from build123d import *

# Parameters (mm, degrees)
SKETCH_W        = 34
SKETCH_H        = 30
PAD_DEPTH       = 22
SKETCH001_R     = 5.5
POCKET_DEPTH    = 30.001
SKETCH002_R     = 2
POCKET001_DEPTH = 22.001
CHAMFER_SIZE    = 3
SKETCH003_R     = 7.5
POCKET002_DEPTH = 24
POCKET003_DEPTH = 3.5


with BuildPart() as part:
    # Sketch → Pad (new body)
    with BuildSketch(Plane.XY):
        with Locations((17, 15)):
            Rectangle(SKETCH_W, SKETCH_H)
    extrude(amount=PAD_DEPTH)

    # Sketch001 (on Face1 of Pad) → Pocket (cut, through all)
    with BuildSketch(Plane.XZ):
        with Locations((17, 11)):
            Circle(SKETCH001_R)
        with BuildLine():
            ThreePointArc((17, 22), (6.777476, 15.062019), (9.450166, 3))
            Line((0, 3), (9.450166, 3))
            Line((0, 22), (0, 3))
            Line((17, 22), (0, 22))
        make_face()
        with BuildLine():
            ThreePointArc((24.549834, 3), (27.222524, 15.062019), (17, 22))
            Line((17, 22), (34, 22))
            Line((34, 22), (34, 3))
            Line((34, 3), (24.549834, 3))
        make_face()
    extrude(amount=-POCKET_DEPTH, mode=Mode.SUBTRACT)

    # Sketch002 (on Face2 of Pocket) → Pocket001 (cut, through all)
    with BuildSketch(Plane(origin=(0, 0, 0), x_dir=(1, 0, 0), z_dir=(0, 0, -1))):
        with Locations((5, -6)):
            Circle(SKETCH002_R)
        with Locations((29, -6)):
            Circle(SKETCH002_R)
        with Locations((29, -24)):
            Circle(SKETCH002_R)
        with Locations((5, -24)):
            Circle(SKETCH002_R)
    extrude(amount=-POCKET001_DEPTH, mode=Mode.SUBTRACT)

    # Chamfer
    chamfer_edges = [part.edges().sort_by_distance(p)[0] for p in [
        (34, 0, 1.5),
        (34, 30, 1.5),
        (0, 30, 1.5),
        (0, 0, 1.5),
    ]]
    chamfer(chamfer_edges, length=CHAMFER_SIZE)

    # Sketch003 (on Face1 of Chamfer) → Pocket002 (cut)
    with BuildSketch(Plane.XZ):
        with Locations((17, 11)):
            Circle(SKETCH003_R)
    extrude(amount=-POCKET002_DEPTH, mode=Mode.SUBTRACT)

    # Sketch004 (on Face6 of Pocket002) → Pocket003 (cut)
    with BuildSketch(Plane.XY.offset(3)):
        Polygon((5, 28.041452), (1.5, 26.020726), (1.5, 21.979274), (5, 19.958548), (8.5, 21.979274), (8.5, 26.020726), align=None)
        Polygon((32.5, 26.020726), (29, 28.041452), (25.5, 26.020726), (25.5, 21.979274), (29, 19.958548), (32.5, 21.979274), align=None)
        Polygon((32.5, 8.020726), (29, 10.041452), (25.5, 8.020726), (25.5, 3.979274), (29, 1.958548), (32.5, 3.979274), align=None)
        Polygon((5, 10.041452), (1.5, 8.020726), (1.5, 3.979274), (5, 1.958548), (8.5, 3.979274), (8.5, 8.020726), align=None)
    extrude(amount=POCKET003_DEPTH, mode=Mode.SUBTRACT)


solid = part.part
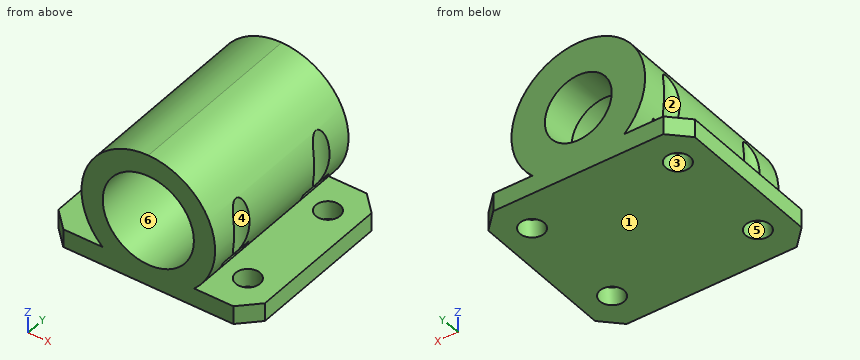
The model under review builds one solid part; all positions refer to its coordinate system, in mm. Face numbers are marked on the shaded views. A direction names the side the tool comes from. Give positions to 0.01 mm unless a question says otherwise; leave off trailing zeros. Order: outer loops, then holes, each group sorted by start corner. A loop starts at its lowest first (then second) coordinate and runs counter-clockwise, first axis right, second up. Notation, with made-up numbers: (52.5, 21) -> (84.5, 21) arc R18 ccw to (84.5, 35) -> close; hole circle Ø7 at (47.5, 39.5). An arc over 180 degrees is marked (long way). Write item = value, one per line. Start each with the question number.
(1) For pin 1 Ø1 at (x, y) = (24.5, 10) entering from -Z; pin 2 Ø1 at (x, y) = (30, 15) entering from +Z; pin 3 Ø4.5 at (x, y) = (5, 6) entering from +Z; pin 4 Ø3 at (x, y) = (5, 24) entering from -Z, all flat-tipped, find the tip position at first contact; note any pin that passes through.
(2) For L1, parallel to Y at x = 29, z = 0.7; L2, parallel to X at y = 6, z = 1.2; L3, parallel to Y at x = 27.5, z = 9.5, list the stretches that pass through material, from the lowest coordinate up. Write a range as from..to.
(3) Tool access review of the marked faces 5 and 6: name each direction out of +Z, -Z, +X, -X, +Y, -Y from which nothing blocks a thin tool from reaching the whole face with its end or side.
(4) Take a section at D-D (x = 29). Write out the cut boundary in (y, z).
(5) Take a section at A-A (x = 4). Write out the cut boundary in (y, z).
(6) Take a section at C-C (y = 12). Write out the cut boundary in (x, z), plus the area to 3 significant figures.
(7) Take a section at B-B (z = 11). Write out the cut boundary in (x, y).
(8) Draft analysis for pull direction X (two halves, no side actions). For the marked faces 1, 2, 3 and 4, state which applies: +X half, -X half, draft (parallel to the pull), parting line (faces both ways), or undercut.
Returned:
q1.pin_1 = 0
q1.pin_2 = 3
q1.pin_3 = 16.09
q1.pin_4 = through
q2.L1 = 0..4, 8..22, 26..30
q2.L2 = 0..3, 7..27, 31..34
q2.L3 = 0..4.68, 7.32..22.68, 25.32..30
q3.face_5 = +Z, -Z
q3.face_6 = -Y
q4.outline = (0, 0) -> (4, 0) -> (4, 3) -> (0, 3) -> close; (8, 0) -> (22, 0) -> (22, 3) -> (8, 3) -> close; (26, 0) -> (30, 0) -> (30, 3) -> (26, 3) -> close
q5.outline = (0, 0) -> (4.27, 0) -> (4.27, 3) -> (0, 3) -> close; (7.73, 0) -> (22.27, 0) -> (22.27, 3) -> (7.73, 3) -> close; (25.73, 0) -> (30, 0) -> (30, 3) -> (25.73, 3) -> close
q6.outline = (0, 0) -> (34, 0) -> (34, 3) -> (24.55, 3) arc R11 ccw (long way) to (9.45, 3) -> (0, 3) -> close; hole circle Ø15 at (17, 11)
q6.area = 274 mm²
q7.outline = (6, 0) -> (9.5, 0) -> (9.5, 24) -> (11.5, 24) -> (11.5, 30) -> (6, 30) -> (6, 25.73) arc R2 cw to (6, 22.27) -> (6, 7.73) arc R2 cw to (6, 4.27) -> close; (22.5, 24) -> (24.5, 24) -> (24.5, 0) -> (28, 0) -> (28, 4.27) arc R2 cw to (28, 7.73) -> (28, 22.27) arc R2 cw to (28, 25.73) -> (28, 30) -> (22.5, 30) -> close
q8.face_1 = draft
q8.face_2 = -X half
q8.face_3 = undercut
q8.face_4 = +X half
